Geometry: final body of the model. Coordinates: model frame, mm. Face numbers are marked on the shaded views. A direction names the side the tool comes from. Round coordinates to 2 decimals unless told otherwise and drop trailing zeros. Loops run counter-clockwise (first coordinate to the right, second up) from the corner with the lowest first, then second, coordinate; pieces in that order, holes last. Notation, with made-up numbers: (-39, 50.5) -> (4, 50.5) arc R14 cw to (4, 75.5) -> close; hole circle Ø1 at (70, -3). An arc over 180 degrees is marked (long way). Answer in a Markdown table with one row per item.
```python
from build123d import *

# Parameters (mm, degrees)
ENLEV_MAT_EXTRU1_DEPTH = 1.1
ESQUISSE3_W            = 1.25
ESQUISSE3_H            = 6
CHANFREIN1_SIZE        = 0.25


with BuildPart() as part:
    # Esquisse1 → Base-Révolution (revolve)
    with BuildSketch(Plane(origin=(0, 0, 0), x_dir=(1, 0, 0), z_dir=(0, 1, 0)), mode=Mode.PRIVATE) as base_r_volution_sk:
        with BuildLine():
            Line((0, 0), (2.25, 0))
            Line((2.25, 0), (2.25, 1.17))
            ThreePointArc((2.25, 1.17), (2.211923882, 1.261923882), (2.12, 1.3))
            Line((2.12, 1.3), (0, 1.3))
            Line((0, 1.3), (0, 0))
        make_face()
    revolve(base_r_volution_sk.sketch.rotate(Axis((0, 0, 0), (0, 0, -1)), 180), axis=Axis((0, 0, 0), (0, 0, -1)))

    # Esquisse2 → enlev-mat-Extru1 (cut)
    with BuildSketch(Plane.XY.offset(-1.3)):
        Polygon((1, -0.577350269), (1, 0.577350269), (0, 1.154700538), (-1, 0.577350269), (-1, -0.577350269), (0, -1.154700538), align=None)
    extrude(amount=ENLEV_MAT_EXTRU1_DEPTH, mode=Mode.SUBTRACT)

    # Esquisse3 → Boss.-Révol.1 (revolve)
    with BuildSketch(Plane(origin=(0, 0, 0), x_dir=(1, 0, 0), z_dir=(0, 1, 0))):
        with Locations((0.625, -3)):
            Rectangle(ESQUISSE3_W, ESQUISSE3_H)
    revolve(axis=Axis((0, 0, 0), (0, 0, 1)))

    # Chanfrein1
    chanfrein1_edges = [part.edges().sort_by_distance(p)[0] for p in [
        (-1.25, 0, 6),
    ]]
    chamfer(chanfrein1_edges, length=CHANFREIN1_SIZE)


solid = part.part
```
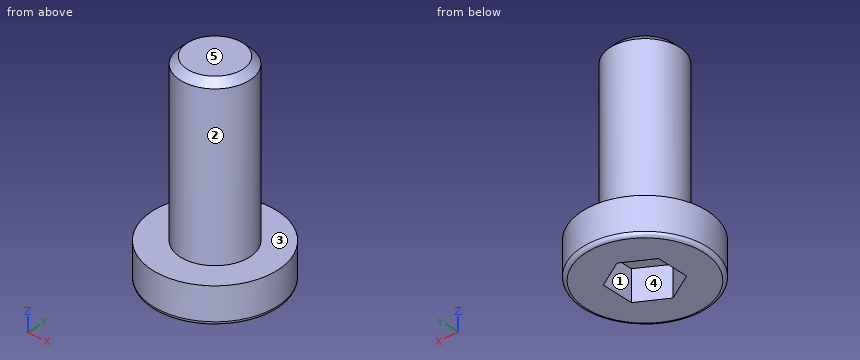
Item 1: Section query A-A, the plane y = 0. Output: boundary loops of the cut face in (x, z), and give its area (3 significant figures).
Ans:
| item | result |
|---|---|
| outline | (-2.25, -1.17) arc R0.13 ccw to (-2.12, -1.3) -> (-1, -1.3) -> (-1, -0.2) -> (1, -0.2) -> (1, -1.3) -> (2.12, -1.3) arc R0.13 ccw to (2.25, -1.17) -> (2.25, 0) -> (1.25, 0) -> (1.25, 5.75) -> (1, 6) -> (-1, 6) -> (-1.25, 5.75) -> (-1.25, 0) -> (-2.25, 0) -> close |
| area | 18.6 mm2 |
Item 2: Set-up query: the marked faces 4 and 5. Return all of +Z, -Z, +X, -X, +Y, -Y with unobstructed straight access to the full face (end or side cutting, diameter ignored); none if empty.
Ans:
| item | result |
|---|---|
| face 4 | -Z |
| face 5 | +Z, +X, -X, +Y, -Y |
Item 3: First-contact query: P1, Ø1.5, axis at y = 1.5, z = 2, coming from the +X side; P2, Ø0.6, axis at x = -0.5, y = 0, coming from the -Z side; P3, Ø1.5, axis at x = 0.5, z = 2.5, coming from the +Y side. Flat tips, straight axial feed; report the tip coordinate or a pass-through.
Ans:
| item | result |
|---|---|
| P1 | x = 1 |
| P2 | z = -0.2 |
| P3 | y = 1.25 |
Item 4: Section query B-B, the plane z = 1.75. Output: boundary loops of the cut face in (x, y).
Ans:
| item | result |
|---|---|
| outline | circle Ø2.5 at (0, 0) |
Item 5: Ray query, L1, parallel to Z at x = -0.4, y = -0.2; L2, parallel to Z at x = -1.25, y = 1.25; L3, parallel to Y at x = 0.55, z = 4.75. Return the intervals inside material, ascending.
Ans:
| item | result |
|---|---|
| L1 | -0.2 to 6 |
| L2 | -1.3 to 0 |
| L3 | -1.12 to 1.12 |
Item 6: Mould query, pull axis X, two halves, no side actions, for the marked faces 1, 2 and 3. Classes: released by +X, released by -X, zero draft, split by the parting line, or undercut.
Ans:
| item | result |
|---|---|
| face 1 | undercut |
| face 2 | split by the parting line |
| face 3 | zero draft |
